```python
from build123d import *

# Parameters (mm, degrees)
SKETCH2_W           = 10
SKETCH2_H           = 10
SKETCH2_W_2         = 8
SKETCH2_H_2         = 8
BOSS_EXTRUDE1_DEPTH = 280
SKETCH3_R           = 1.5
CUT_EXTRUDE1_DEPTH  = 28


with BuildPart() as part:
    # Sketch2 → Boss-Extrude1 (new body)
    with BuildSketch(Plane.XY):
        Rectangle(SKETCH2_W, SKETCH2_H)
        Rectangle(SKETCH2_W_2, SKETCH2_H_2, mode=Mode.SUBTRACT)
    extrude(amount=BOSS_EXTRUDE1_DEPTH)

    # Sketch3 → Cut-Extrude1 (cut)
    with BuildSketch(Plane(origin=(0, 5, 0), x_dir=(1, 0, 0), z_dir=(0, 1, 0))):
        with Locations((0, -15)):
            Circle(SKETCH3_R)
        with Locations((0, -30)):
            Circle(SKETCH3_R)
        with Locations((0, -265)):
            Circle(SKETCH3_R)
        with Locations((0, -250)):
            Circle(SKETCH3_R)
    extrude(amount=-CUT_EXTRUDE1_DEPTH, mode=Mode.SUBTRACT)


solid = part.part
```
The listing builds one solid part. Answer for the finished solid, in the listing's coordinates (mm). A direction names the side the tool comes from. Coordinates: 2 decimals unless noted, no trailing zeros. Loops run counter-clockwise (first coordinate to the right, second up) from the corner with the lowest first, then second, coordinate; pieces in that order, holes last. Notation, with made-up numbers: (67, 37) -> (94, 37) arc R33 cw to (94, 72) -> close; hole circle Ø5 at (56.25, -3.5). An arc over 180 degrees is marked (long way). Use one line per item in the form item = value. Start each with the question number.
Item 1: The part is cut by section C-C on x = 0. Count the separate pieces of the cut face and the enclosed holes in it, then the cut area to 3 significant figures.
Item 2: The part is cut by section B-B on z = 78. Determine the outline of the cut face in (x, y).
Item 3: A tool of negligible diameter and unlimited length cuts with its end or side. For faces 4 (the face through (-4.5, 0.1, 0)), 5 (the face through (0, -4, 138)), from which of +Z, -Z, +X, -X, +Y, -Y can it reach the whole face along a straight path? Write none if from no direction.
Item 4: The part is cut by section A-A on y = 2.5. Determine the outline of the cut face in (x, z).
Item 5: The mould has two halves that part along Y. Classify faces 1 (the face through (-4, 0, 138)), 2 (the face through (0, 5, 138)), 3 (the face through (-4.5, 0.1, 280)): released by +Y, released by -Y, zero draft, split by the parting line, or undercut.
Item 6: Consider L1, parallel to Z at x = 0, y = -4.7; L2, parallel to Y at x = 3.25, z = 176; L3, parallel to X at y = 4.65, z = 30. Determine where each line is inside the solid, lowest interval first. Write a range as [from, to].
Answer key:
q1.separate_pieces = 10
q1.enclosed_holes = 0
q1.area = 536 mm2
q2.outline = (-5, -5) -> (5, -5) -> (5, 5) -> (-5, 5) -> close; hole (-4, -4) -> (4, -4) -> (4, 4) -> (-4, 4) -> close
q3.face_4 = -Z, +X, -X, +Y, -Y
q3.face_5 = +Z, -Z
q4.outline = (-5, 0) -> (-4, 0) -> (-4, 280) -> (-5, 280) -> close; (4, 0) -> (5, 0) -> (5, 280) -> (4, 280) -> close
q5.face_1 = undercut
q5.face_2 = released by +Y
q5.face_3 = zero draft
q6.L1 = [0, 13.5], [16.5, 28.5], [31.5, 248.5], [251.5, 263.5], [266.5, 280]
q6.L2 = [-5, -4], [4, 5]
q6.L3 = [-5, -1.5], [1.5, 5]
